Read the model definition and answer for the solid it produces. Units are mm, in the model's axes. A direction names the side the tool comes from. Coordinates: 2 decimals unless noted, no trailing zeros. Loops run counter-clockwise (first coordinate to the right, second up) from the corner with the lowest first, then second, coordinate; pieces in that order, holes last. Notation, with made-up numbers: (64.25, -21.75) -> (123.25, -21.75) arc R24 cw to (123.25, 3.25) -> close; hole circle Ø1 at (18.5, 64). An arc over 180 degrees is marked (long way). Answer in a Markdown table with one row per item.
```python
from build123d import *

# Parameters (mm, degrees)
SKETCH013_W     = 31.8
SKETCH013_H     = 31.8
SKETCH013_R     = 1.75
SKETCH013_W_2   = 27.700439
SKETCH013_H_2   = 2
PAD005_DEPTH    = 1
SKETCH014_W     = 31.8
SKETCH014_H     = 31.8
SKETCH014_W_2   = 27.700439
SKETCH014_H_2   = 27.4
PAD006_DEPTH    = 32.4
SKETCH024_W     = 5.5
SKETCH024_H     = 27
POCKET010_DEPTH = 2
SKETCH025_W     = 27
SKETCH025_H     = 5.5
POCKET011_DEPTH = 1.5
SKETCH026_W     = 27
SKETCH026_H     = 5.5
POCKET012_DEPTH = 1.5


with BuildPart() as part:
    # Sketch013 (on Face2 of Binder003) → Pad005 (new body)
    with BuildSketch(Plane.XZ.offset(-33.95)):
        with Locations((13.749781, 0.8)):
            Rectangle(SKETCH013_W, SKETCH013_H)
        with Locations((5.24978, 9.3)):
            Circle(SKETCH013_R, mode=Mode.SUBTRACT)
        with Locations((22.24978, 9.3)):
            Circle(SKETCH013_R, mode=Mode.SUBTRACT)
        with Locations((22.24978, -7.7)):
            Circle(SKETCH013_R, mode=Mode.SUBTRACT)
        with Locations((5.24978, -7.7)):
            Circle(SKETCH013_R, mode=Mode.SUBTRACT)
        with Locations((13.74978, 0.8)):
            Rectangle(SKETCH013_W_2, SKETCH013_H_2, mode=Mode.SUBTRACT)
    extrude(amount=PAD005_DEPTH)

    # Sketch014 (on Face14 of Pad005) → Pad006 (join)
    with BuildSketch(Plane.XZ.offset(-32.95)):
        with Locations((13.74978, 0.8)):
            Rectangle(SKETCH014_W, SKETCH014_H)
        with Locations((13.74978, 0)):
            Rectangle(SKETCH014_W_2, SKETCH014_H_2, mode=Mode.SUBTRACT)
    extrude(amount=PAD006_DEPTH)

    # Sketch024 (on Face14 of Pad006) → Pocket010 (cut)
    with BuildSketch(Plane.XY.offset(16.7)):
        with Locations((13.74978, 14.05)):
            Rectangle(SKETCH024_W, SKETCH024_H)
    extrude(amount=-POCKET010_DEPTH, mode=Mode.SUBTRACT)

    # Sketch025 (on Face2 of Pocket010) → Pocket011 (cut)
    with BuildSketch(Plane(origin=(-2.15022, 0, 0), x_dir=(0, -1, 0), z_dir=(-1, 0, 0))):
        with Locations((-14.05, 0.8)):
            Rectangle(SKETCH025_W, SKETCH025_H)
    extrude(amount=-POCKET011_DEPTH, mode=Mode.SUBTRACT)

    # Sketch026 (on Face4 of Pocket011) → Pocket012 (cut)
    with BuildSketch(Plane.YZ.offset(29.64978)):
        with Locations((14.05, 0.8)):
            Rectangle(SKETCH026_W, SKETCH026_H)
    extrude(amount=-POCKET012_DEPTH, mode=Mode.SUBTRACT)


solid = part.part
```
1. A cutting plane is placed at A-A on x = 10. Give the vertices of the cut face in (y, z), and give its area (3 significant figures).
A:
| item | result |
|---|---|
| outline | (0.55, -15.1) -> (33.95, -15.1) -> (33.95, -0.2) -> (32.95, -0.2) -> (32.95, -13.7) -> (0.55, -13.7) -> close; (0.55, 13.7) -> (32.95, 13.7) -> (32.95, 1.8) -> (33.95, 1.8) -> (33.95, 16.7) -> (0.55, 16.7) -> close |
| area | 172 mm2 |
2. The mould has two halves that part along Z. Classify faces 6 (the flat face through (14, 17, -15.1)), 7 (the flat face through (-0.65, 14, 1)), 8 (the flat face through (14, 33.95, -3)), 9 (the flat face through (14, 32.95, 8)): pulls with the +Z half, pulls with the -Z half, needs draft (parallel to the pull), parting line crosses it, or undercut.
A:
| item | result |
|---|---|
| face 6 | pulls with the -Z half |
| face 7 | undercut |
| face 8 | needs draft |
| face 9 | undercut |
3. Given pin 1 Ø2 at (x, z) = (13, 16) entering from -Y; pin 2 Ø9.5 at (x, z) = (9, 7.5) entering from -Y; pin 3 Ø1.7 at (x, y) = (13.5, 17) entering from +Z, each flat-ended and moving along its own axis, determine where each tip first touches the part or whether it passes through.
A:
| item | result |
|---|---|
| pin 1 | stops at y = 27.55 |
| pin 2 | stops at y = 32.95 |
| pin 3 | stops at z = 14.7 |
4. Find the intervals of material crossed by probe 1 along Z at (x, y) = (21, 22); probe 2 along X at (y, z) = (19, 10); probe 3 along X at (y, z) = (13, 2), in increasing order.
A:
| item | result |
|---|---|
| probe 1 | z = -15.1 to -13.7, 13.7 to 16.7 |
| probe 2 | x = -2.15 to -0.1, 27.6 to 29.65 |
| probe 3 | x = -0.65 to -0.1, 27.6 to 28.15 |
5. A tool of negligible diameter and unlimited length cuts with its end or side. For faces 1 (the flat face through (29, 14, 3.55)), 2 (the flat face through (-1, 14, -1.95)), 3 (the flat face through (13.6, 33.5, 1.8)), 4 (the flat face through (11, 14, 16)), 5 (the flat face through (14, 32.95, -7)), from which of +Z, -Z, +X, -X, +Y, -Y can it reach the whole face along a straight path? Write none if from no direction.
A:
| item | result |
|---|---|
| face 1 | +X, -Y |
| face 2 | -X, -Y |
| face 3 | +Y, -Y |
| face 4 | +Z, -Y |
| face 5 | -Y |
6. A cutting plane is placed at C-C on y = 11. Give the vertices of the cut face in (x, z), and give its area (3 significant figures).
A:
| item | result |
|---|---|
| outline | (-2.15, -15.1) -> (29.65, -15.1) -> (29.65, -1.95) -> (28.15, -1.95) -> (28.15, 3.55) -> (29.65, 3.55) -> (29.65, 16.7) -> (16.5, 16.7) -> (16.5, 14.7) -> (11, 14.7) -> (11, 16.7) -> (-2.15, 16.7) -> (-2.15, 3.55) -> (-0.65, 3.55) -> (-0.65, -1.95) -> (-2.15, -1.95) -> close; hole (-0.1, -13.7) -> (27.6, -13.7) -> (27.6, 13.7) -> (-0.1, 13.7) -> close |
| area | 225 mm2 |
7. A cutting plane is placed at B-B on z = -7.7. Count the separate pieces of the cut face and the enclosed holes in it, and give its area (3 significant figures).
A:
| item | result |
|---|---|
| separate pieces | 3 |
| enclosed holes | 0 |
| area | 158 mm2 |
